```python
from build123d import *

# Parameters (mm, degrees)
SKETCH1_W                       = 50
SKETCH1_H                       = 95
BOSS_EXTRUDE1_DEPTH             = 2.25
M2_5_CLEARANCE_HOLE1_AT_2_COUNT = 2
M2_5_CLEARANCE_HOLE1_AT_2_PITCH = 15.5
M2_5_CLEARANCE_HOLE1_AT_3_COUNT = 2
M2_5_CLEARANCE_HOLE1_AT_3_PITCH = 21.920310217
M2_5_CLEARANCE_HOLE1_AT_4_COUNT = 2
M2_5_CLEARANCE_HOLE1_AT_4_PITCH = 15.5
SKETCH4_W                       = 50
SKETCH4_H                       = 5
CUT_EXTRUDE1_DEPTH              = 54.865573421
CUT_EXTRUDE2_DEPTH              = 2.25
M4_CLEARANCE_HOLE1_D            = 4.3
M4_CLEARANCE_HOLE1_DEPTH        = 10.1
M4_CLEARANCE_HOLE1_TIP          = 1.291850331
FILLET1_R                       = 3.1524
M2_5_CLEARANCE_HOLE2_D          = 2.9


with BuildPart() as part:
    # Sketch1 → Boss-Extrude1 (new, symmetric)
    with BuildSketch(Plane(origin=(0, 0, 0), x_dir=(1, 0, 0), z_dir=(0, 1, 0))):
        Rectangle(SKETCH1_W, SKETCH1_H)
    extrude(amount=BOSS_EXTRUDE1_DEPTH, both=True)

    # Sketch3 → M2.5 Clearance Hole1 (revolve, cut)
    with BuildSketch(Plane(origin=(2.15, 2.25, 20.15), x_dir=(0, 0, 1), z_dir=(1, 0, 0))):
        Polygon((0, 0), (0, 7.161161836), (1.35, 6.35), (1.35, 0), align=None)
    m2_5_clearance_hole1 = revolve(axis=Axis((2.15, 8.6, 20.15), (0, -1, 0)), mode=Mode.SUBTRACT)

    # M2.5 Clearance Hole1 at 2: M2.5 Clearance Hole1 ×2
    with Locations(*[(0, 0, i * M2_5_CLEARANCE_HOLE1_AT_2_PITCH) for i in range(1, M2_5_CLEARANCE_HOLE1_AT_2_COUNT)]):
        add(m2_5_clearance_hole1, mode=Mode.SUBTRACT)

    # M2.5 Clearance Hole1 at 3: M2.5 Clearance Hole1 ×2
    with Locations(*[Vector(-0.7071067811865477, 0, 0.7071067811865475) * (i * M2_5_CLEARANCE_HOLE1_AT_3_PITCH) for i in range(1, M2_5_CLEARANCE_HOLE1_AT_3_COUNT)]):
        add(m2_5_clearance_hole1, mode=Mode.SUBTRACT)

    # M2.5 Clearance Hole1 at 4: M2.5 Clearance Hole1 ×2
    with Locations(*[(-i * M2_5_CLEARANCE_HOLE1_AT_4_PITCH, 0, 0) for i in range(1, M2_5_CLEARANCE_HOLE1_AT_4_COUNT)]):
        add(m2_5_clearance_hole1, mode=Mode.SUBTRACT)

    # Sketch4 → Cut-Extrude1 (cut, through all)
    with BuildSketch(Plane(origin=(0, 2.25, 0), x_dir=(1, 0, 0), z_dir=(0, 1, 0))):
        with Locations((0, -45)):
            Rectangle(SKETCH4_W, SKETCH4_H)
    cut_extrude1 = extrude(amount=-CUT_EXTRUDE1_DEPTH, mode=Mode.SUBTRACT)

    # Mirror1: M2.5 Clearance Hole1, Cut-Extrude1 across plane
    add(m2_5_clearance_hole1.mirror(Plane.XY), mode=Mode.SUBTRACT)
    add(cut_extrude1.mirror(Plane.XY), mode=Mode.SUBTRACT)

    # Mirror1 copy 1 sketch → Mirror1 copy 1 (revolve, cut)
    with BuildSketch(Plane(origin=(2.15, 2.25, -35.65), x_dir=(0, 0, -1), z_dir=(1, 0, 0))):
        Polygon((0, 0), (0, -7.161161836), (1.35, -6.35), (1.35, 0), align=None)
    revolve(axis=Axis((2.15, 8.6, -35.65), (0, 1, 0)), mode=Mode.SUBTRACT)

    # Mirror1 copy 2 sketch → Mirror1 copy 2 (revolve, cut)
    with BuildSketch(Plane(origin=(-13.35, 2.25, -35.65), x_dir=(0, 0, -1), z_dir=(1, 0, 0))):
        Polygon((0, 0), (0, -7.161161836), (1.35, -6.35), (1.35, 0), align=None)
    revolve(axis=Axis((-13.35, 8.6, -35.65), (0, 1, 0)), mode=Mode.SUBTRACT)

    # Mirror1 copy 3 sketch → Mirror1 copy 3 (revolve, cut)
    with BuildSketch(Plane(origin=(-13.35, 2.25, -20.15), x_dir=(0, 0, -1), z_dir=(1, 0, 0))):
        Polygon((0, 0), (0, -7.161161836), (1.35, -6.35), (1.35, 0), align=None)
    revolve(axis=Axis((-13.35, 8.6, -20.15), (0, 1, 0)), mode=Mode.SUBTRACT)

    # Sketch5 → Cut-Extrude2 (cut)
    with BuildSketch(Plane(origin=(0, 2.25, 0), x_dir=(1, 0, 0), z_dir=(0, 1, 0))):
        with BuildLine():
            Line((25, -36.6524), (16, -36.6524))
            ThreePointArc((16, -36.6524), (13.770916583, -35.729083417), (12.8476, -33.5))
            Line((12.8476, -33.5), (12.8476, -27.5))
            ThreePointArc((12.8476, -27.5), (13.770916583, -25.270916583), (16, -24.3476))
            Line((16, -24.3476), (25, -24.3476))
            Line((25, -24.3476), (25, -36.6524))
        make_face()
        with BuildLine():
            Line((25, 6.1524), (25, -6.1524))
            Line((25, -6.1524), (16, -6.1524))
            ThreePointArc((16, -6.1524), (13.770916583, -5.229083417), (12.8476, -3))
            Line((12.8476, -3), (12.8476, 3))
            ThreePointArc((12.8476, 3), (13.770916583, 5.229083417), (16, 6.1524))
            Line((16, 6.1524), (25, 6.1524))
        make_face()
        with BuildLine():
            Line((25, 36.6524), (25, 24.3476))
            Line((25, 24.3476), (16, 24.3476))
            ThreePointArc((16, 24.3476), (13.770916583, 25.270916583), (12.8476, 27.5))
            Line((12.8476, 27.5), (12.8476, 33.5))
            ThreePointArc((12.8476, 33.5), (13.770916583, 35.729083417), (16, 36.6524))
            Line((16, 36.6524), (25, 36.6524))
        make_face()
    extrude(amount=-CUT_EXTRUDE2_DEPTH, mode=Mode.SUBTRACT)

    # M4 Clearance Hole1
    with Locations(Plane(origin=(0, 0, 0), x_dir=(1, 0, 0), z_dir=(0, 1, 0))):
        with Locations((19.3048, -30.5), (19.3048, 0), (19.3048, 30.5)):
            Hole(M4_CLEARANCE_HOLE1_D / 2, depth=M4_CLEARANCE_HOLE1_DEPTH)
            with Locations((0, 0, -(M4_CLEARANCE_HOLE1_DEPTH + M4_CLEARANCE_HOLE1_TIP / 2))):  # 118° drill point
                Cone(0, M4_CLEARANCE_HOLE1_D / 2, M4_CLEARANCE_HOLE1_TIP, mode=Mode.SUBTRACT)

    # Fillet1
    fillet1_edges = [part.edges().sort_by_distance(p)[0] for p in [
        (25, 1.125, 24.3476),
        (25, 1.125, 36.6524),
        (25, 1.125, 6.1524),
        (25, 1.125, -6.1524),
        (25, 1.125, -24.3476),
        (25, 1.125, -36.6524),
    ]]
    fillet(fillet1_edges, radius=FILLET1_R)

    # M2.5 Clearance Hole2 (through all)
    with Locations(Plane(origin=(0, -2.25, 0), x_dir=(-1, 0, 0), z_dir=(0, -1, 0))):
        with Locations((19.641987941, 6), (19.641987941, -6)):
            Hole(M2_5_CLEARANCE_HOLE2_D / 2)


solid = part.part
```
Could you check a few things on this model? Use its own coordinates, in mm. A direction names the side the tool comes from. Round coordinates to 2 decimals unless told otherwise and drop trailing zeros. Write each loop counter-clockwise with the first axis right and the second up, starting at its lowest first coordinate (ties: lowest second). Pieces come first, ordered by that corner, then holes. Notation, with made-up numbers: M 12,-21.5 L 66,-21.5 A10 cw 66,-14.5 Z; hole C 12,-20.5 d3. An arc over 180 degrees is marked long. Answer in a Markdown table with one row per item. Add a question column.
Q1. Imagine slicing it at B-B (z = 30.5). Please give me the cut outline in (x, y), then the cut area to 3 significant figures.
Q2. On a 3-axis mill with a long thin cutter (end or side, diameter ignored), from which of +Z, -Z, +X, -X, +Y, -Y can I reach the whole of each face in a straight line? I mean faces 4 (the flat face through (25, -0.5, 0.6)), 5 (the flat face through (12.848, 1, 31)). Say none if no direction works.
Q3. Imagine slicing it at D-D (y = -1.35). Give the number of separate pieces and of enclosed holes in the cut face, then the cut area to 3 significant figures.
Q4. If we mould it in two halves opening along X, with no side actions, what happens to faces 1 (the cylindrical face through (-18.26, 0.03, -6.44)), 2 (the flat face through (19, 1, -24.348)), 3 (the cylindrical face through (13.796, 1.141, -25.247))? For each: +X half, -X half, draft (parallel to the pull), parting line (faces both ways), or undercut.
Q5. Will these pins go through, and if not, where does the flat tip stop? pin 1 Ø3 at (x, z) = (2.15, 20.15) entering from -Y; pin 2 Ø5 at (x, z) = (19.3, 30.5) entering from +Y; pin 3 Ø1.1 at (y, z) = (1.5, 0.5) entering from +X.
Q6. If I drill on line 1 (Z direction, x = -13.35, y = 0.5); line 2 (X direction, y = -0.75, z = 20.15); line 3 (X direction, y = 0.5, z = 1), over which ranges is the centre line in solid material (lowest first)? Write a range as from..to.
Q7. Imagine slicing it at C-C (z = -20.15). Please give me the cut outline in (x, y).
Q8. Imagine slicing it at A-A (x = 2.15). Please give me the cut outline in (y, z), then the cut area to 3 significant figures.
Values:
| question | item | result |
|---|---|---|
| 1 | outline | M -25,-2.25 L 17.15,-2.25 L 17.15,0 L 12.85,0 L 12.85,2.25 L -25,2.25 Z; M 21.45,-2.25 L 25,-2.25 L 25,0 L 21.45,0 Z |
| 1 | area | 188 mm^2 |
| 2 | face 4 | +Z, -Z, +X, +Y, -Y |
| 2 | face 5 | +X, +Y |
| 3 | separate pieces | 1 |
| 3 | enclosed holes | 13 |
| 3 | area | 4,150 mm^2 |
| 4 | face 1 | undercut |
| 4 | face 2 | draft |
| 4 | face 3 | +X half |
| 5 | pin 1 | y = -2.25 |
| 5 | pin 2 | y = 0 |
| 5 | pin 3 | x = 12.85 |
| 6 | line 1 | -42.5..-37, -34.3..-21.5, -18.8..18.8, 21.5..34.3, 37..42.5 |
| 6 | line 2 | -25..-14.7, -12..0.8, 3.5..25 |
| 6 | line 3 | -25..12.85 |
| 7 | outline | M -25,-2.25 L -14.7,-2.25 L -14.7,2.25 L -25,2.25 Z; M -12,-2.25 L 0.8,-2.25 L 0.8,2.25 L -12,2.25 Z; M 3.5,-2.25 L 25,-2.25 L 25,2.25 L 3.5,2.25 Z |
| 8 | outline | M -2.25,-42.5 L 2.25,-42.5 L 2.25,-37 L -2.25,-37 Z; M -2.25,-34.3 L 2.25,-34.3 L 2.25,-21.5 L -2.25,-21.5 Z; M -2.25,-18.8 L 2.25,-18.8 L 2.25,18.8 L -2.25,18.8 Z; M -2.25,21.5 L 2.25,21.5 L 2.25,34.3 L -2.25,34.3 Z; M -2.25,37 L 2.25,37 L 2.25,42.5 L -2.25,42.5 Z |
| 8 | area | 334 mm^2 |
